Work out the finished part from the listing and answer in its coordinate system (mm). A direction names the side the tool comes from. Give positions to 0.01 mm unless a question says otherwise; leave off trailing zeros. Loops run counter-clockwise (first coordinate to the right, second up) from the corner with the lowest first, then second, coordinate; pieces in that order, holes last. Notation, with made-up numbers: M 62,39 L 93,39 A24 cw 93,74 Z; hole C 61,29.25 d2. An arc over 180 degrees is marked long. Use a Markdown table: item, result.
```python
from build123d import *

# Parameters (mm, degrees)
SKETCH_1_R          = 3.1
SKETCH_1_R_2        = 1.4
EXTRUDE_1_DEPTH     = 3
FILLET_1_R          = 15
CUT_EXTRUDE_1_DEPTH = 10
FILLET_2_R          = 2


with BuildPart() as part:
    # 草图1 → 凸台-拉伸1 (new body)
    with BuildSketch(Plane.XY):
        Polygon((20.145101954, 130.106797695), (-10, 108.335377566), (-10, 0), (-10, -46), (36, -46), (120.145101954, -46), (120.145101954, 130.106797695), align=None)
        Circle(SKETCH_1_R, mode=Mode.SUBTRACT)
        with Locations((26, 122)):
            Circle(SKETCH_1_R, mode=Mode.SUBTRACT)
        with Locations((36, -36)):
            Circle(SKETCH_1_R, mode=Mode.SUBTRACT)
        with Locations((28.145101954, 50.106797695)):
            Circle(SKETCH_1_R_2, mode=Mode.SUBTRACT)
        with Locations((72.145101954, 50.106797695)):
            Circle(SKETCH_1_R_2, mode=Mode.SUBTRACT)
        with Locations((16.395101954, -5.893202305)):
            Circle(SKETCH_1_R_2, mode=Mode.SUBTRACT)
        with Locations((83.895101954, -5.893202305)):
            Circle(SKETCH_1_R_2, mode=Mode.SUBTRACT)
        with BuildLine():
            Line((30.145101954, 110.106797695), (70.145101954, 110.106797695))
            ThreePointArc((70.145101954, 110.106797695), (80.145101954, 100.106797695), (70.145101954, 90.106797695))
            Line((70.145101954, 90.106797695), (30.145101954, 90.106797695))
            ThreePointArc((30.145101954, 90.106797695), (20.145101954, 100.106797695), (30.145101954, 110.106797695))
        make_face(mode=Mode.SUBTRACT)
    extrude(amount=EXTRUDE_1_DEPTH)

    # 圆角1
    fillet_1_edges = [part.edges().sort_by_distance(p)[0] for p in [
        (-10, -46, 1.5),
        (-10, 108.335377566, 1.5),
        (20.145101954, 130.106797695, 1.5),
        (120.145101954, 130.106797695, 1.5),
        (120.145101954, -46, 1.5),
    ]]
    fillet(fillet_1_edges, radius=FILLET_1_R)

    # 草图2 → 切除-拉伸1 (cut)
    with BuildSketch(Plane.XY.offset(3)):
        Polygon((9.95669343, -11.893202305), (114.145101954, -26.979143214), (114.145101954, -11.893202305), align=None)
        Polygon((-4, -13.914059091), (-4, -29), (100.188408524, -29), align=None)
        Polygon((23.784683113, 0.106797695), (33.01682597, 44.106797695), (67.273377938, 44.106797695), (76.505520795, 0.106797695), align=None)
        Polygon((14.742218034, 10.577914397), (23.665689084, 53.106797695), (-1.853126388, 53.106797695), align=None)
        Polygon((-4, 7), (11.844621313, 7), (-4, 47.605005448), align=None)
        Polygon((111.910718161, 53.106797695), (76.624514825, 53.106797695), (87.082812907, 3.262994069), align=None)
        Polygon((114.145101954, 0.106797695), (114.145101954, 48.621111695), (89.979434332, 0.106797695), align=None)
        Polygon((-4, 82.051397551), (-4, 58.16219784), (46.39985599, 70.106797695), align=None)
        Polygon((4.672694987, 84.106797695), (55.072550977, 72.16219784), (105.472406967, 84.106797695), align=None)
        Polygon((114.145101954, 82.051397551), (63.745245965, 70.106797695), (114.145101954, 58.16219784), align=None)
        Polygon((55.072550977, 68.051397551), (4.672694987, 56.106797695), (105.472406967, 56.106797695), align=None)
        Polygon((87.773796421, 124.106797695), (114.145101954, 93.188715346), (114.145101954, 124.106797695), align=None)
        Polygon((85.145101954, 121.024880044), (85.145101954, 90.106797695), (111.516407487, 90.106797695), align=None)
    extrude(amount=-CUT_EXTRUDE_1_DEPTH, mode=Mode.SUBTRACT)

    # 圆角2
    fillet_2_edges = [part.edges().sort_by_distance(p)[0] for p in [
        (-4, 58.16219784, 1.5),
        (-4, 82.051397551, 1.5),
        (46.39985599, 70.106797695, 1.5),
        (55.072550977, 72.16219784, 1.5),
        (4.672694987, 84.106797695, 1.5),
        (105.472406967, 84.106797695, 1.5),
        (111.910718161, 53.106797695, 1.5),
        (87.082812907, 3.262994069, 1.5),
        (76.624514825, 53.106797695, 1.5),
        (114.145101954, 48.621111695, 1.5),
        (114.145101954, 0.106797695, 1.5),
        (89.979434332, 0.106797695, 1.5),
        (-4, -13.914059091, 1.5),
        (100.188408524, -29, 1.5),
        (-4, -29, 1.5),
        (23.784683113, 0.106797695, 1.5),
        (33.01682597, 44.106797695, 1.5),
        (67.273377938, 44.106797695, 1.5),
        (76.505520795, 0.106797695, 1.5),
        (-4, 47.605005448, 1.5),
        (11.844621313, 7, 1.5),
        (-4, 7, 1.5),
        (-1.853126388, 53.106797695, 1.5),
        (23.665689084, 53.106797695, 1.5),
        (14.742218034, 10.577914397, 1.5),
        (4.672694987, 56.106797695, 1.5),
        (55.072550977, 68.051397551, 1.5),
        (105.472406967, 56.106797695, 1.5),
        (63.745245965, 70.106797695, 1.5),
        (114.145101954, 82.051397551, 1.5),
        (114.145101954, 58.16219784, 1.5),
        (85.145101954, 121.024880044, 1.5),
        (111.516407487, 90.106797695, 1.5),
        (85.145101954, 90.106797695, 1.5),
        (87.773796421, 124.106797695, 1.5),
        (114.145101954, 124.106797695, 1.5),
        (114.145101954, 93.188715346, 1.5),
        (9.95669343, -11.893202305, 1.5),
        (114.145101954, -11.893202305, 1.5),
        (114.145101954, -26.979143214, 1.5),
    ]]
    fillet(fillet_2_edges, radius=FILLET_2_R)


solid = part.part
```
(1) A cutting plane is placed at B-B (y = 32). Write down the section's boundary in (x, z), and give its area (3 significant figures).
Entries:
| item | result |
|---|---|
| outline | M -10,0 L -4,0 L -4,3 L -10,3 Z; M 2.09,0 L 6.38,0 L 6.38,3 L 2.09,3 Z; M 19.24,0 L 30.48,0 L 30.48,3 L 19.24,3 Z; M 69.81,0 L 81.05,0 L 81.05,3 L 69.81,3 Z; M 101.4,0 L 105.87,0 L 105.87,3 L 101.4,3 Z; M 114.15,0 L 120.15,0 L 120.15,3 L 114.15,3 Z |
| area | 130 mm² |
(2) The mould has two halves that part along X. Classify faces 3 (the flat face through (99.914, 29.022, 1.521)), 4 (the flat face through (19.59, 33.69, 1.52)), 5 (the cylindrical face through (115.634, 125.829, 1.521)), 6 (the flat face through (69, 43, 0)): released by +X, released by -X, zero draft, split by the parting line, or undercut.
Entries:
| item | result |
|---|---|
| face 3 | undercut |
| face 4 | undercut |
| face 5 | released by +X |
| face 6 | zero draft |
(3) Which of the six approach directions +Z, -Z, +X, -X, +Y, -Y give full straight-line access (tool end or side, diameter ignored) to faces 1 (the cylindrical face through (20.148, 99.887, 1.479)), 2 (the cylindrical face through (-5.72, -41.49, 1.52))?
Entries:
| item | result |
|---|---|
| face 1 | +Z, -Z |
| face 2 | +Z, -Z, -X, -Y |
(4) A cutting plane is placed at A-A (y = -36). Write down the section's boundary in (x, z).
Entries:
| item | result |
|---|---|
| outline | M -9.14,0 L 32.9,0 L 32.9,3 L -9.14,3 Z; M 39.1,0 L 119.29,0 L 119.29,3 L 39.1,3 Z |
(5) A cutting plane is placed at C-C (x = 101.5). Write down the section's boundary in (y, z), and give its area (3 significant figures).
Entries:
| item | result |
|---|---|
| outline | M -46,0 L -25.15,0 L -25.15,3 L -46,3 Z; M -11.89,0 L 0.11,0 L 0.11,3 L -11.89,3 Z; M 23.24,0 L 32.21,0 L 32.21,3 L 23.24,3 Z; M 53.11,0 L 61.16,0 L 61.16,3 L 53.11,3 Z; M 79.05,0 L 90.11,0 L 90.11,3 L 79.05,3 Z; M 101.85,0 L 108.01,0 L 108.01,3 L 101.85,3 Z; M 124.11,0 L 130.11,0 L 130.11,3 L 124.11,3 Z |
| area | 219 mm² |
(6) A cutting plane is placed at D-D (z = 1.7). Count the separate pieces of the cut face and the enclosed holes in it, and give its area (3 significant figures).
Entries:
| item | result |
|---|---|
| separate pieces | 1 |
| enclosed holes | 21 |
| area | 12,500 mm² |
(7) Consider probe 1 along X at (y, z) = (48, 1.05); probe 2 along X at (y, z) = (26.5, 0.2); probe 3 along X at (y, z) = (71.5, 1.25). Determine where each line is inside the solid, lowest interval first. Write a range as [from, to].
Entries:
| item | result |
|---|---|
| probe 1 | x = [-10, 0.14], [22.59, 77.7], [109.37, 120.15] |
| probe 2 | x = [-10, -4], [4.24, 8.53], [18.08, 29.32], [70.97, 82.21], [98.66, 103.13], [114.15, 120.15] |
| probe 3 | x = [-10, -4], [39.16, 70.98], [114.15, 120.15] |
(8) Given P1, Ø1.7, axis at x = 72.15, y = 50.11, coming from the +Z side, flat-ended and moving along its own axis, determine where the tip first touches the part or whether it passes through.
Entries:
| item | result |
|---|---|
| P1 | passes through |
